Model file for the job. Use its own axes, mm. A direction names the side the tool comes from. Give positions to 0.01 mm unless a question says otherwise; leave off trailing zeros. Write each loop counter-clockwise with the first axis right and the second up, starting at its lowest first coordinate (ties: lowest second). Pieces come first, ordered by that corner, then holes. Notation, with made-up numbers: M 83.25,83 L 136.25,83 A23 cw 136.25,122 Z; hole C 2.25,72.25 d6. An arc over 180 degrees is marked long. Answer as a JSON object with one key per item and string values. Group by question number.
```python
from build123d import *

# Parameters (mm, degrees)
SALIENTE_EXTRUIR1_DEPTH = 580
REDONDEO1_R             = 5
CORTAR_EXTRUIR1_REACH   = 585.866
CROQUIS2_R              = 5


with BuildPart() as part:
    # Croquis1 → Saliente-Extruir1 (new body)
    with BuildSketch(Plane(origin=(0, 0, 0), x_dir=(0, 0, -1), z_dir=(1, 0, 0))):
        Polygon((10, 0), (0, 10), (0, 29), (8, 29), (8, 45), (0, 45), (0, 60), (38, 60), (38, 0), align=None)
    extrude(amount=SALIENTE_EXTRUIR1_DEPTH)

    # Redondeo1
    redondeo1_edges = [part.edges().sort_by_distance(p)[0] for p in [
        (290, 0, -38),
    ]]
    fillet(redondeo1_edges, radius=REDONDEO1_R)

    # Croquis2 → Cortar-Extruir1 (cut, up to next)
    with BuildSketch(Plane.XY.offset(-8), mode=Mode.PRIVATE) as cortar_extruir1_sk1:
        with Locations((25, 37)):
            Circle(CROQUIS2_R)
    cortar_extruir1_tool1 = extrude(cortar_extruir1_sk1.sketch, amount=-CORTAR_EXTRUIR1_REACH, mode=Mode.PRIVATE) & part.part
    # Croquis2 → Cortar-Extruir1 (cut, up to next)
    with BuildSketch(Plane.XY.offset(-8), mode=Mode.PRIVATE) as cortar_extruir1_sk2:
        with Locations((157.5, 37)):
            Circle(CROQUIS2_R)
    cortar_extruir1_tool2 = extrude(cortar_extruir1_sk2.sketch, amount=-CORTAR_EXTRUIR1_REACH, mode=Mode.PRIVATE) & part.part
    # Croquis2 → Cortar-Extruir1 (cut, up to next)
    with BuildSketch(Plane.XY.offset(-8), mode=Mode.PRIVATE) as cortar_extruir1_sk3:
        with Locations((555, 37)):
            Circle(CROQUIS2_R)
    cortar_extruir1_tool3 = extrude(cortar_extruir1_sk3.sketch, amount=-CORTAR_EXTRUIR1_REACH, mode=Mode.PRIVATE) & part.part
    # Croquis2 → Cortar-Extruir1 (cut, up to next)
    with BuildSketch(Plane.XY.offset(-8), mode=Mode.PRIVATE) as cortar_extruir1_sk4:
        with Locations((290, 37)):
            Circle(CROQUIS2_R)
    cortar_extruir1_tool4 = extrude(cortar_extruir1_sk4.sketch, amount=-CORTAR_EXTRUIR1_REACH, mode=Mode.PRIVATE) & part.part
    # Croquis2 → Cortar-Extruir1 (cut, up to next)
    with BuildSketch(Plane.XY.offset(-8), mode=Mode.PRIVATE) as cortar_extruir1_sk5:
        with Locations((422.5, 37)):
            Circle(CROQUIS2_R)
    cortar_extruir1_tool5 = extrude(cortar_extruir1_sk5.sketch, amount=-CORTAR_EXTRUIR1_REACH, mode=Mode.PRIVATE) & part.part
    add(cortar_extruir1_tool1.solids().sort_by_distance((25, 37, -8))[0], mode=Mode.SUBTRACT)
    add(cortar_extruir1_tool2.solids().sort_by_distance((157.5, 37, -8))[0], mode=Mode.SUBTRACT)
    add(cortar_extruir1_tool3.solids().sort_by_distance((555, 37, -8))[0], mode=Mode.SUBTRACT)
    add(cortar_extruir1_tool4.solids().sort_by_distance((290, 37, -8))[0], mode=Mode.SUBTRACT)
    add(cortar_extruir1_tool5.solids().sort_by_distance((422.5, 37, -8))[0], mode=Mode.SUBTRACT)


solid = part.part
```
Q1. Wall check: L1, parallel to Y at x = 157, z = -30; L2, parallel to Z at x = 403.5, y = 41; L3, parallel to Z at x = 318.5, y = 7.5. Give the ranges that are in metal, low to high.
Q2. Slice it at B-B, the plane y = 37. Write the cut outline in (x, z), then the cut area to 3 significant figures.
Q3. Slice it at C-C, the plane x = 240. Write the cut outline in (y, z).
Q4. Drop flat-ended pins along their axis: P1, Ø10, axis at x = 117, y = 35.5, coming from the +Z side; P2, Ø4, axis at x = 409, z = -3, coming from the -Y side. Give the stop position or say it passes through.
Q5. Two-plate mould, pull along Y, no slides. Class faces 3 (the flat face through (286, 0, -22)), 4 (the cylindrical face through (559.619, 35.085, -22.79)), 5 (the flat face through (0, 30, -19)): +Y half, -Y half, draft (parallel to the pull), parting line (faces both ways), or undercut.
Q6. Slice it at A-A, the plane x = 422.5. Write the cut outline in (y, z), then the cut area to 3 significant figures.
Q7. 3-axis set-ups, long thin cutter, end or side, ignore diameter. For faces 1 (the cylindrical face through (21, 40, -23)), 2 (the flat face through (285.9, 40.4, -8)): which of +Z, -Z, +X, -X, +Y, -Y reach the whole face in a straight line?
Solved:
{
 "1": {"L1": "y = 0 to 32.03, 41.97 to 60", "L2": "z = -38 to -8", "L3": "z = -38 to -2.5"},
 "2": {"outline": "M 0,-38 L 20,-38 L 20,-8 L 0,-8 Z; M 30,-38 L 152.5,-38 L 152.5,-8 L 30,-8 Z; M 162.5,-38 L 285,-38 L 285,-8 L 162.5,-8 Z; M 295,-38 L 417.5,-38 L 417.5,-8 L 295,-8 Z; M 427.5,-38 L 550,-38 L 550,-8 L 427.5,-8 Z; M 560,-38 L 580,-38 L 580,-8 L 560,-8 Z", "area": "15,900 mm²"},
 "3": {"outline": "M 0,-33 A5 ccw 5,-38 L 60,-38 L 60,0 L 45,0 L 45,-8 L 29,-8 L 29,0 L 10,0 L 0,-10 Z"},
 "4": {"P1": "stops at z = -8", "P2": "stops at y = 5"},
 "5": {"face 3": "-Y half", "face 4": "undercut", "face 5": "draft"},
 "6": {"outline": "M 0,-33 A5 ccw 5,-38 L 32,-38 L 32,-8 L 29,-8 L 29,0 L 10,0 L 0,-10 Z; M 42,-38 L 60,-38 L 60,0 L 45,0 L 45,-8 L 42,-8 Z", "area": "1,800 mm²"},
 "7": {"face 1": "+Z, -Z", "face 2": "+Z, +X, -X"}
}
